from build123d import *

# Parameters (mm, degrees)
SKETCH1_W                     = 18.25
SKETCH1_H                     = 12.88
BOSS_EXTRUDE1_DEPTH           = 5.89
SKETCH2_W                     = 3.79
SKETCH2_H                     = 3.9
CUT_EXTRUDE1_DEPTH            = 9
SKETCH3_W                     = 3
SKETCH3_H                     = 3.11
BOSS_EXTRUDE2_DEPTH           = 1.41
CUT_EXTRUDE2_DEPTH            = 3
SKETCH5_W                     = 1.23
SKETCH5_H                     = 1.23
CUT_EXTRUDE3_DEPTH            = 4
SKETCH8_W                     = 1.23
SKETCH8_H                     = 1.23
SKETCH9_W                     = 1
SKETCH9_H                     = 3.11
BOSS_EXTRUDE3_DEPTH           = 0.25
BOSS_EXTRUDE5_DEPTH           = 1.5875
BOSS_EXTRUDE6_DEPTH           = 1.46
BOSS_EXTRUDE6_DRAFT           = 28
BOSS_EXTRUDE6_PROFILE_2_DEPTH = 1.46
BOSS_EXTRUDE6_PROFILE_2_DRAFT = 28
BOSS_EXTRUDE6_PROFILE_3_DEPTH = 1.46
BOSS_EXTRUDE6_PROFILE_3_DRAFT = 28
BOSS_EXTRUDE6_PROFILE_4_DEPTH = 1.46
BOSS_EXTRUDE6_PROFILE_4_DRAFT = 28


with BuildPart() as part:
    # Sketch1 → Boss-Extrude1 (new body)
    with BuildSketch(Plane(origin=(0, 0, 0), x_dir=(1, 0, 0), z_dir=(0, 1, 0))):
        with Locations((9.125, 6.44)):
            Rectangle(SKETCH1_W, SKETCH1_H)
    extrude(amount=BOSS_EXTRUDE1_DEPTH)

    # Sketch2 → Cut-Extrude1 (cut)
    with BuildSketch(Plane.XY):
        with Locations((2.765, 3.21048567)):
            Rectangle(SKETCH2_W, SKETCH2_H)
        Polygon((5.12, 5.16048567), (8.91, 5.16048567), (8.91, 2.26048567), (7.91, 1.26048567), (6.12, 1.26048567), (5.12, 2.26048567), align=None)
        with Locations((11.265, 3.21048567)):
            Rectangle(SKETCH2_W, SKETCH2_H)
        with Locations((15.515, 3.21048567)):
            Rectangle(SKETCH2_W, SKETCH2_H)
    extrude(amount=-CUT_EXTRUDE1_DEPTH, mode=Mode.SUBTRACT)

    # Sketch3 → Boss-Extrude2 (add)
    with BuildSketch(Plane(origin=(0, 5.89, 0), x_dir=(1, 0, 0), z_dir=(0, 1, 0))):
        with Locations((9, 1.555)):
            Rectangle(SKETCH3_W, SKETCH3_H)
    extrude(amount=BOSS_EXTRUDE2_DEPTH)

    # Sketch4 → Cut-Extrude2 (cut)
    with BuildSketch(Plane.ZY.offset(-7.5)):
        Polygon((-2.258367839, 7.3), (0, 5.89), (0, 7.3), align=None)
    extrude(amount=-CUT_EXTRUDE2_DEPTH, mode=Mode.SUBTRACT)

    # Sketch5 → Cut-Extrude3 (cut)
    with BuildSketch(Plane(origin=(0, 0, -12.88), x_dir=(-1, 0, 0), z_dir=(0, 0, -1))):
        with Locations((-2.785, 2.645)):
            Rectangle(SKETCH5_W, SKETCH5_H)
        with Locations((-6.990239219, 2.642823938)):
            Rectangle(SKETCH5_W, SKETCH5_H)
        with Locations((-11.195478439, 2.640647876)):
            Rectangle(SKETCH5_W, SKETCH5_H)
        with Locations((-15.400717658, 2.638471814)):
            Rectangle(SKETCH5_W, SKETCH5_H)
    extrude(amount=-CUT_EXTRUDE3_DEPTH, mode=Mode.SUBTRACT)

    # Sweep2: sweep along a path in Sketch7
    with BuildLine(Plane.ZY) as sweep2_path:
        Line((-4.3, 2.72), (-12.700459496, 2.72))
        ThreePointArc((-12.700459496, 2.72), (-13.534520585, 2.374520585), (-13.88, 1.540459496))
        Line((-13.88, 1.540459496), (-13.88, -3.3375))
    # Sketch8 → Sweep2 (sweep)
    with BuildSketch(Plane.XZ.offset(3.3375)):
        with Locations((15.397064507, -13.830209109)):
            Rectangle(SKETCH8_W, SKETCH8_H)
        with Locations((11.191825288, -13.832385171)):
            Rectangle(SKETCH8_W, SKETCH8_H)
        with Locations((6.986586068, -13.834561233)):
            Rectangle(SKETCH8_W, SKETCH8_H)
        with Locations((2.781346849, -13.836737294)):
            Rectangle(SKETCH8_W, SKETCH8_H)
    sweep(path=sweep2_path.line)

    # Sketch9 → Boss-Extrude3 (add)
    with BuildSketch(Plane(origin=(0, 5.89, 0), x_dir=(1, 0, 0), z_dir=(0, 1, 0))):
        with Locations((15.5, 1.555)):
            Rectangle(SKETCH9_W, SKETCH9_H)
    extrude(amount=BOSS_EXTRUDE3_DEPTH)

    # Sketch10 → Boss-Extrude5 (add)
    with BuildSketch(Plane.XZ):
        with BuildLine():
            Line((2.55, -5.735786438), (2.55, -8.564213562))
            ThreePointArc((2.55, -8.564213562), (1.55, -7.15), (2.55, -5.735786438))
        make_face()
        with BuildLine():
            Line((3.55, -5.735786438), (3.55, -8.564213562))
            ThreePointArc((3.55, -8.564213562), (4.55, -7.15), (3.55, -5.735786438))
        make_face()
        with BuildLine():
            Line((14.7, -5.735786438), (14.7, -8.564213562))
            ThreePointArc((14.7, -8.564213562), (13.7, -7.15), (14.7, -5.735786438))
        make_face()
        with BuildLine():
            Line((15.7, -5.735786438), (15.7, -8.564213562))
            ThreePointArc((15.7, -8.564213562), (16.7, -7.15), (15.7, -5.735786438))
        make_face()
    extrude(amount=BOSS_EXTRUDE5_DEPTH)


with BuildPart() as boss_extrude6_tool:
    # Sketch12 → Boss-Extrude6 (with draft: the straight prism first)
    with BuildSketch(Plane.XZ.offset(1.5875)):
        with BuildLine():
            ThreePointArc((2.55, -5.735786438), (0.266263579, -7.15), (2.55, -8.564213562))
            Line((2.55, -8.564213562), (2.55, -5.735786438))
        make_face()
    extrude(amount=BOSS_EXTRUDE6_DEPTH)
    # Boss-Extrude6: the draft: its side faces are tilted about the plane it starts from
    boss_extrude6_sides = [boss_extrude6_tool.faces().sort_by_distance(p)[0] for p in [
        (2.55, -2.3175, -7.15),
        (0.266263579, -2.3175, -7.15),
    ]]
    draft(boss_extrude6_sides, Plane.XZ.offset(1.5875), BOSS_EXTRUDE6_DRAFT)


with BuildPart() as part_1:
    add(part.part)

    # Boss-Extrude6: add boss_extrude6_tool
    add(boss_extrude6_tool.part)


with BuildPart() as boss_extrude6_profile_2_tool:
    # Sketch12 → Boss-Extrude6 profile 2 (with draft: the straight prism first)
    with BuildSketch(Plane.XZ.offset(1.5875)):
        with BuildLine():
            Line((3.55, -5.735786438), (3.55, -8.564213562))
            ThreePointArc((3.55, -8.564213562), (5.833736421, -7.15), (3.55, -5.735786438))
        make_face()
    extrude(amount=BOSS_EXTRUDE6_PROFILE_2_DEPTH)
    # Boss-Extrude6 profile 2: the draft: its side faces are tilted about the plane it starts from
    boss_extrude6_profile_2_sides = [boss_extrude6_profile_2_tool.faces().sort_by_distance(p)[0] for p in [
        (3.55, -2.3175, -7.15),
        (5.833736421, -2.3175, -7.15),
    ]]
    draft(boss_extrude6_profile_2_sides, Plane.XZ.offset(1.5875), BOSS_EXTRUDE6_PROFILE_2_DRAFT)


with BuildPart() as part_2:
    add(part_1.part)

    # Boss-Extrude6 profile 2: add boss_extrude6_profile_2_tool
    add(boss_extrude6_profile_2_tool.part)


with BuildPart() as boss_extrude6_profile_3_tool:
    # Sketch12 → Boss-Extrude6 profile 3 (with draft: the straight prism first)
    with BuildSketch(Plane.XZ.offset(1.5875)):
        with BuildLine():
            ThreePointArc((14.7, -5.735786438), (12.416263579, -7.15), (14.7, -8.564213562))
            Line((14.7, -8.564213562), (14.7, -5.735786438))
        make_face()
    extrude(amount=BOSS_EXTRUDE6_PROFILE_3_DEPTH)
    # Boss-Extrude6 profile 3: the draft: its side faces are tilted about the plane it starts from
    boss_extrude6_profile_3_sides = [boss_extrude6_profile_3_tool.faces().sort_by_distance(p)[0] for p in [
        (12.416263579, -2.3175, -7.15),
        (14.7, -2.3175, -7.15),
    ]]
    draft(boss_extrude6_profile_3_sides, Plane.XZ.offset(1.5875), BOSS_EXTRUDE6_PROFILE_3_DRAFT)


with BuildPart() as part_3:
    add(part_2.part)

    # Boss-Extrude6 profile 3: add boss_extrude6_profile_3_tool
    add(boss_extrude6_profile_3_tool.part)


with BuildPart() as boss_extrude6_profile_4_tool:
    # Sketch12 → Boss-Extrude6 profile 4 (with draft: the straight prism first)
    with BuildSketch(Plane.XZ.offset(1.5875)):
        with BuildLine():
            Line((15.7, -5.735786438), (15.7, -8.564213562))
            ThreePointArc((15.7, -8.564213562), (17.983736421, -7.15), (15.7, -5.735786438))
        make_face()
    extrude(amount=BOSS_EXTRUDE6_PROFILE_4_DEPTH)
    # Boss-Extrude6 profile 4: the draft: its side faces are tilted about the plane it starts from
    boss_extrude6_profile_4_sides = [boss_extrude6_profile_4_tool.faces().sort_by_distance(p)[0] for p in [
        (15.7, -2.3175, -7.15),
        (17.983736421, -2.3175, -7.15),
    ]]
    draft(boss_extrude6_profile_4_sides, Plane.XZ.offset(1.5875), BOSS_EXTRUDE6_PROFILE_4_DRAFT)


with BuildPart() as part_4:
    add(part_3.part)

    # Boss-Extrude6 profile 4: add boss_extrude6_profile_4_tool
    add(boss_extrude6_profile_4_tool.part)


solid = part_4.part
Check sheet for the modelled part. Datum: model origin and axes. Units: mm. A direction names the side the tool comes from. Give positions to 0.01 mm unless a question says otherwise; leave off trailing zeros. Order: outer loops, then holes, each group sorted by start corner. A loop starts at its lowest first (then second) coordinate and runs counter-clockwise, first axis right, second up. Notation, with made-up numbers: (62.25, 52) - (115.25, 52) arc R16 cw to (115.25, 56) - close; hole circle Ø4 at (30, -20). An arc over 180 degrees is marked (long way). Answer as CSV lines item,"result".
1. Section check A-A (z = -7.15). State how many separate pieces and enclosed holes the cut face has, then the cut area to 3 significant figures.
Result sheet:
separate pieces,"5"
enclosed holes,"4"
area,"70.6 mm²"
2. Section check B-B (y = 0.75). Record the boundary of the cut face in (x, z).
Result sheet:
outline,"(0, -12.88) - (18.25, -12.88) - (18.25, 0) - (0, 0) - close; (2.17, -14.45) - (3.4, -14.45) - (3.4, -13.22) - (2.17, -13.22) - close; (6.37, -14.45) - (7.6, -14.45) - (7.6, -13.22) - (6.37, -13.22) - close; (10.58, -14.45) - (11.81, -14.45) - (11.81, -13.22) - (10.58, -13.22) - close; (14.78, -14.45) - (16.01, -14.45) - (16.01, -13.22) - (14.78, -13.22) - close"
3. Go/stop test with flat-tipped pins: P1, Ø0.8, axis at y = -0.5, z = -7, coming from the +X side; P2, Ø1.5, axis at x = 14, z = -7.5, coming from the +Y side; P3, Ø3, axis at x = 11.5, y = -1, coming from the -Z side. Record where each tip stops, or that it passes through.
Result sheet:
P1,"x = 16.7"
P2,"y = 5.89"
P3,"z = -14.45"
4. Tool access check on faces 1 (the face through (17.41, 3, -4)), 2 (the face through (2.55, -1, -7)), 3 (the face through (8.98, 6.6, -1.14)), 4 (the face through (14.317, -2.307, -7.17)). Record the directions out of +Z, -Z, +X, -X, +Y, -Y that give a thin tool (end or side, any length) a straight path to the whole face; none if there is none.
Result sheet:
face 1,"+Z"
face 2,"+Z, -Y"
face 3,"+Z, -X, +Y"
face 4,"+Z, -Z, -Y"
5. Mould release check, pull along Y, two halves, no side actions. Record for faces 5 (the face through (9, 7.3, -2.7)), 6 (the face through (11, 1.26, -4)), 7 (the face through (10.5, 6.4, -1.9)): released by +Y, released by -Y, zero draft, split by the parting line, or undercut.
Result sheet:
face 5,"released by +Y"
face 6,"undercut"
face 7,"zero draft"
6. Scan lines: probe 1 along X at (y, z) = (4.5, -4.75); probe 2 along Y at (x, z) = (2.75, -7.5); probe 3 along Y at (x, z) = (10.5, -7.5). Record each from-to range of solid material in increasing order. Write a range as from..to.
Result sheet:
probe 1,"0..0.87, 4.66..5.12, 8.91..9.37, 13.16..13.62, 17.41..18.25"
probe 2,"0..1.26, 2.06..3.29, 5.16..5.89"
probe 3,"0..1.26, 5.16..5.89"
